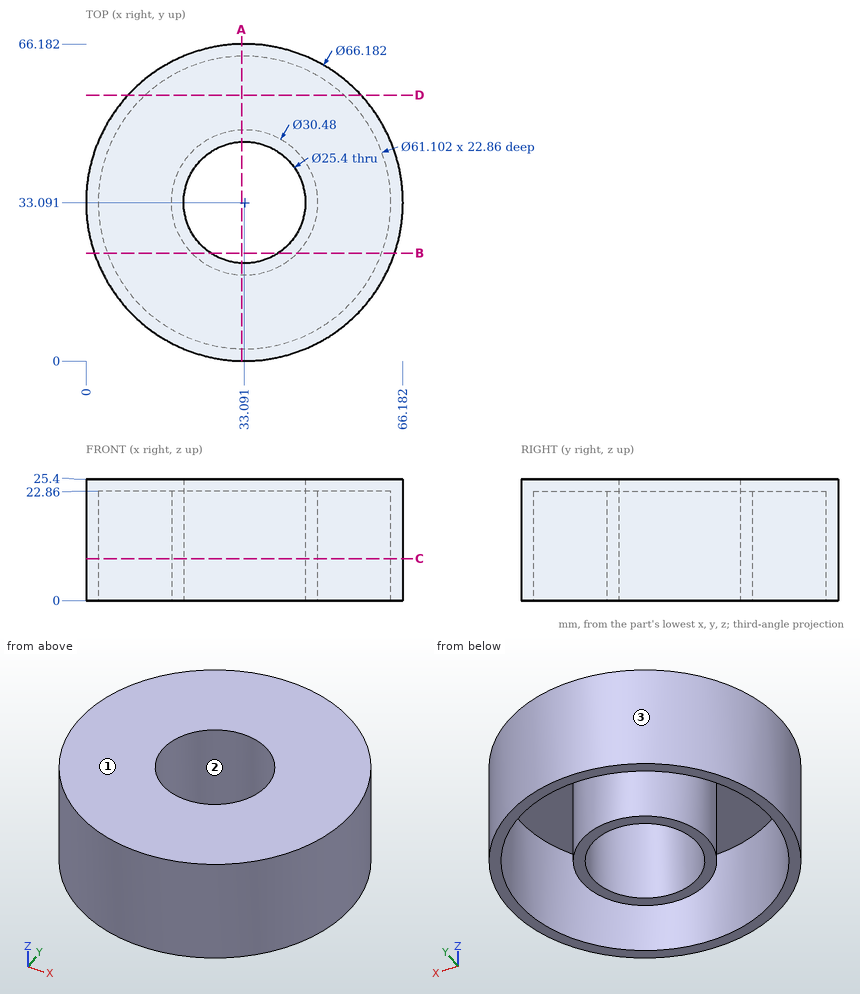
Job drawing, mm, ordinate dimensions from the low corner. One solid piece. Give positions to 0.01 mm unless a question says otherwise; leave off trailing zeros. Write each loop counter-clockwise with the first axis right and the second up, starting at its lowest first coordinate (ties: lowest second). Pieces come first, ordered by that corner, then holes. Notation, with made-up numbers: (73.25, -37.75) -> (89.25, -37.75) arc R20 ccw to (89.25, -23.75) -> close; hole circle Ø9 at (28.25, 8.5). An arc over 180 degrees is marked (long way). Return JSON: item names as keys, results as strings.
Item 1: Drill centre lines: probe 1 along X at (y, z) = (33, 1.75); probe 2 along X at (y, z) = (46, 14.5); probe 3 along Y at (x, z) = (40, 5.75) (1 decimal). Where is each one in solid material? Low to high.
Answer below:
{"probe 1": "x = 0 to 2.54, 17.85 to 20.39, 45.79 to 48.33, 63.64 to 66.18", "probe 2": "x = 2.62 to 5.4, 24.99 to 41.19, 60.78 to 63.56", "probe 3": "y = 0.7 to 3.3, 19.5 to 22.4, 43.7 to 46.7, 62.9 to 65.5"}
Item 2: Band-saw the part on A-A (x = 32.5). List the corners of the cut face in (y, z).
Answer below:
{"outline": "(0.01, 0) -> (2.55, 0) -> (2.55, 22.86) -> (17.86, 22.86) -> (17.86, 0) -> (20.4, 0) -> (20.4, 25.4) -> (0.01, 25.4) -> close; (45.78, 0) -> (48.32, 0) -> (48.32, 22.86) -> (63.64, 22.86) -> (63.64, 0) -> (66.18, 0) -> (66.18, 25.4) -> (45.78, 25.4) -> close"}
Item 3: Two-plate mould, pull along X, no slides. Class the marked faces 1, 2 and 3: +X half, -X half, draft (parallel to the pull), parting line (faces both ways), or undercut.
Answer below:
{"face 1": "draft", "face 2": "undercut", "face 3": "parting line"}
Item 4: Drop flat-ended pins along their axis: pin 1 (3 mm diameter, centred on x = 50.5, z = 4.5, fed in from -Y) (3 decimals); pin 2 (12 mm diameter, centred on x = 40.5, z = 18, fed in from +Y); pin 3 (4 mm diameter, centred on x = 24.5, y = 14.5, fed in from -Z). Give the stop position or say it passes through.
Answer below:
{"pin 1": "stops at y = 4.075", "pin 2": "stops at y = 66.15", "pin 3": "stops at z = 22.86"}
Item 5: Band-saw the part on D-D (y = 55.5). List the corners of the cut face in (x, z).
Answer below:
{"outline": "(8.74, 0) -> (12.33, 0) -> (12.33, 22.86) -> (53.86, 22.86) -> (53.86, 0) -> (57.44, 0) -> (57.44, 25.4) -> (8.74, 25.4) -> close"}
Item 6: Band-saw the part on B-B (y = 22.5). List the corners of the cut face in (x, z), then the cut area to 3 significant figures.
Answer below:
{"outline": "(1.74, 0) -> (4.43, 0) -> (4.43, 22.86) -> (22.13, 22.86) -> (22.13, 0) -> (26.08, 0) -> (26.08, 25.4) -> (1.74, 25.4) -> close; (40.1, 0) -> (44.05, 0) -> (44.05, 22.86) -> (61.75, 22.86) -> (61.75, 0) -> (64.44, 0) -> (64.44, 25.4) -> (40.1, 25.4) -> close", "area": "427 mm2"}
Item 7: Band-saw the part on C-C (z = 8.75). List the corners of the cut face in (x, y), then the cut area to 3 significant figures.
Answer below:
{"outline": "circle Ø66.18 at (33.09, 33.09); circle Ø30.48 at (33.09, 33.09); hole circle Ø61.1 at (33.09, 33.09); hole circle Ø25.4 at (33.09, 33.09)", "area": "731 mm2"}
